Model file for the job. Use its own axes, mm. Coordinates: 2 decimals unless noted, no trailing zeros. Order: outer loops, then holes, each group sorted by start corner. A loop starts at its lowest first (then second) coordinate and runs counter-clockwise, first axis right, second up. Notation, with made-up numbers: (12, 9.25) -> (65, 9.25) arc R20 cw to (65, 32.25) -> close; hole circle Ø5 at (82, 42.25). An arc over 180 degrees is marked (long way). Return JSON: item names as keys, results as strings. Group by question number.
1) Cut at A-A (z = -215). Write the cut outline in (x, y), and give its area (3 significant figures).
2) Cut at B-B (y = -2.25). State how many separate pieces and enclosed holes the cut face has, and give its area (3 significant figures).
3) Probe line 1 (X direction, y = -3, z = 1); line 2 (X direction, y = -5.65, z = -243); line 3 (Z direction, x = 171, y = -3.5). List the from-to ranges inside material, lowest first.
4) Cut at C-C (z = 76). Write the cut outline in (x, y), and give its area (3 significant figures).
5) Flat gauge pins, fed straight in: pin 1 (5.5 mm diameter, centred on x = 28.99, z = -186.01, fed in from -Y); pin 2 (9 mm diameter, centred on x = 167.87, z = 0, fed in from +Y). Where does each tip first touch, or does it go through?
from build123d import *

# Parameters (mm, degrees)
SKETCH1_R           = 17.5
SKETCH1_R_2         = 3.4
SKETCH1_R_3         = 2.731026391
BOSS_EXTRUDE1_DEPTH = 6
FILLET1_R           = 8
SKETCH5_R           = 3.4
CUT_EXTRUDE4_DEPTH  = 20
CUT_EXTRUDE5_DEPTH  = 10
CUT_EXTRUDE6_DEPTH  = 10
FILLET2_R           = 8
CHAMFER1_SIZE       = 5.15


with BuildPart() as part:
    # Sketch1 → Boss-Extrude1 (new body)
    with BuildSketch(Plane(origin=(0, 0, 0), x_dir=(1, 0, 0), z_dir=(0, 1, 0))):
        Polygon((-175, 275), (-225, -275), (225, -275), (175, 275), align=None)
        with Locations(Location((0, 215, 0), (0, 0, 270))):
            Circle(SKETCH1_R, mode=Mode.SUBTRACT)
        with Locations(Location((-145.777131586, 243, 0), (0, 0, 270))):
            Circle(SKETCH1_R_2, mode=Mode.SUBTRACT)
        with Locations(Location((145.777131586, 243, 0), (0, 0, 90))):
            Circle(SKETCH1_R_2, mode=Mode.SUBTRACT)
        with Locations(Location((-189.958949768, -243, 0), (0, 0, 270))):
            Circle(SKETCH1_R_2, mode=Mode.SUBTRACT)
        with Locations(Location((189.958949768, -243, 0), (0, 0, 90))):
            Circle(SKETCH1_R_2, mode=Mode.SUBTRACT)
        with Locations(Location((-167.868040677, 0, 0), (0, 0, 270))):
            Circle(SKETCH1_R_2, mode=Mode.SUBTRACT)
        with Locations(Location((167.868040677, 0, 0), (0, 0, 90))):
            Circle(SKETCH1_R_2, mode=Mode.SUBTRACT)
        with Locations(Location((0, 115, 0), (0, 0, 270))):
            Circle(SKETCH1_R_3, mode=Mode.SUBTRACT)
    extrude(amount=-BOSS_EXTRUDE1_DEPTH)

    # Fillet1
    fillet1_edges = [part.edges().sort_by_distance(p)[0] for p in [
        (175, -3, -275),
        (225, -3, 275),
        (-225, -3, 275),
        (-175, -3, -275),
    ]]
    fillet(fillet1_edges, radius=FILLET1_R)

    # Sketch5 → Cut-Extrude4 (cut)
    with BuildSketch(Plane(origin=(0, 0, 377.333920735), x_dir=(0, 0, 1), z_dir=(0, 1, 0))):
        with Locations((-563.342542706, 28.991378029)):
            Circle(SKETCH5_R)
        with Locations((-563.342542706, -28.991378029)):
            Circle(SKETCH5_R)
        with Locations((-621.325298763, -28.991378029)):
            Circle(SKETCH5_R)
        with Locations((-621.325298763, 28.991378029)):
            Circle(SKETCH5_R)
    extrude(amount=-CUT_EXTRUDE4_DEPTH, mode=Mode.SUBTRACT)

    # Sketch6 → Cut-Extrude5 (cut)
    with BuildSketch(Plane(origin=(0, 0, 0), x_dir=(1, 0, 0), z_dir=(0, 1, 0))):
        Polygon((-204.631966366, -95.133074099), (-182.722315824, 145.873081867), (-194.245635018, 159.701064899), (-218.459949399, -106.656393293), align=None)
    cut_extrude5 = extrude(amount=-CUT_EXTRUDE5_DEPTH, mode=Mode.SUBTRACT)

    # Sketch7 → Cut-Extrude6 (cut)
    with BuildSketch(Plane(origin=(0, 0, 0), x_dir=(1, 0, 0), z_dir=(0, 1, 0))):
        Polygon((-31.320564901, -271.594250629), (31.320564901, -271.594250629), (45, -279.893229805), (-45, -279.893229805), align=None)
    extrude(amount=-CUT_EXTRUDE6_DEPTH, mode=Mode.SUBTRACT)

    # Mirror2: Cut-Extrude5 across plane
    add(cut_extrude5.mirror(Plane(origin=(0, 0, 0), x_dir=(0, 0, 1), z_dir=(1, 0, 0))), mode=Mode.SUBTRACT)

    # Fillet2
    fillet2_edges = [part.edges().sort_by_distance(p)[0] for p in [
        (-182.722315824, -3, -145.873081867),
        (-204.631966366, -3, 95.133074099),
        (36.934355042, -3, 275),
        (-36.934355042, -3, 275),
        (-31.320564901, -3, 271.594250629),
        (31.320564901, -3, 271.594250629),
        (204.631966366, -3, 95.133074099),
        (182.722315824, -3, -145.873081867),
    ]]
    fillet(fillet2_edges, radius=FILLET2_R)

    # Chamfer1
    chamfer1_edges = [part.edges().sort_by_distance(p)[0] for p in [
        (-145.777131586, 0, -246.4),
        (145.777131586, 0, -239.6),
        (-189.958949768, 0, 239.6),
        (189.958949768, 0, 246.4),
        (-167.868040677, 0, -3.4),
        (167.868040677, 0, 3.4),
    ]]
    chamfer(chamfer1_edges, length=CHAMFER1_SIZE)


solid = part.part
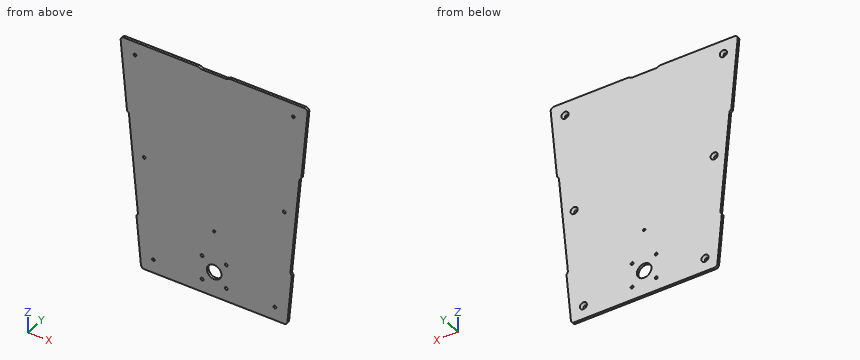
Answers below:
{
 "1": {"outline": "(-180.45, -6) -> (-17.5, -6) -> (-17.5, 0) -> (-180.45, 0) -> close; (17.5, -6) -> (180.45, -6) -> (180.45, 0) -> (17.5, 0) -> close", "area": "1,960 mm^2"},
 "2": {"separate pieces": "1", "enclosed holes": "12", "area": "216,000 mm^2"},
 "3": {"line 1": "x = -196.07 to -173.33, -162.41 to 162.41, 173.33 to 196.07", "line 2": "x = -177.91 to -149.18, -142.38 to -32.24, -25.74 to 25.74, 32.24 to 142.38, 149.18 to 177.91", "line 3": "z = -274.29 to -3.96, 3.96 to 275"},
 "4": {"outline": "(-202.89, -6) -> (202.89, -6) -> (202.89, 0) -> (-202.89, 0) -> close", "area": "2,430 mm^2"},
 "5": {"pin 1": "passes through", "pin 2": "stops at y = -4.05"}
}
